Geometry check sheet. Reference: drawing and pictorial views, mm from the part's lowest x, y, z. A direction names the side the tool comes from. Coordinates: 2 decimals unless noted, no trailing zeros. Loops run counter-clockwise (first coordinate to the right, second up) from the corner with the lowest first, then second, coordinate; pieces in that order, holes last. Notation, with made-up numbers: M 22,-27.5 L 60,-27.5 A18 cw 60,-17.5 Z; hole C 51.5,-7.75 d9. An arc over 180 degrees is marked long. Write each question's results on one line, items separated by ' | '. Start each with the question number.
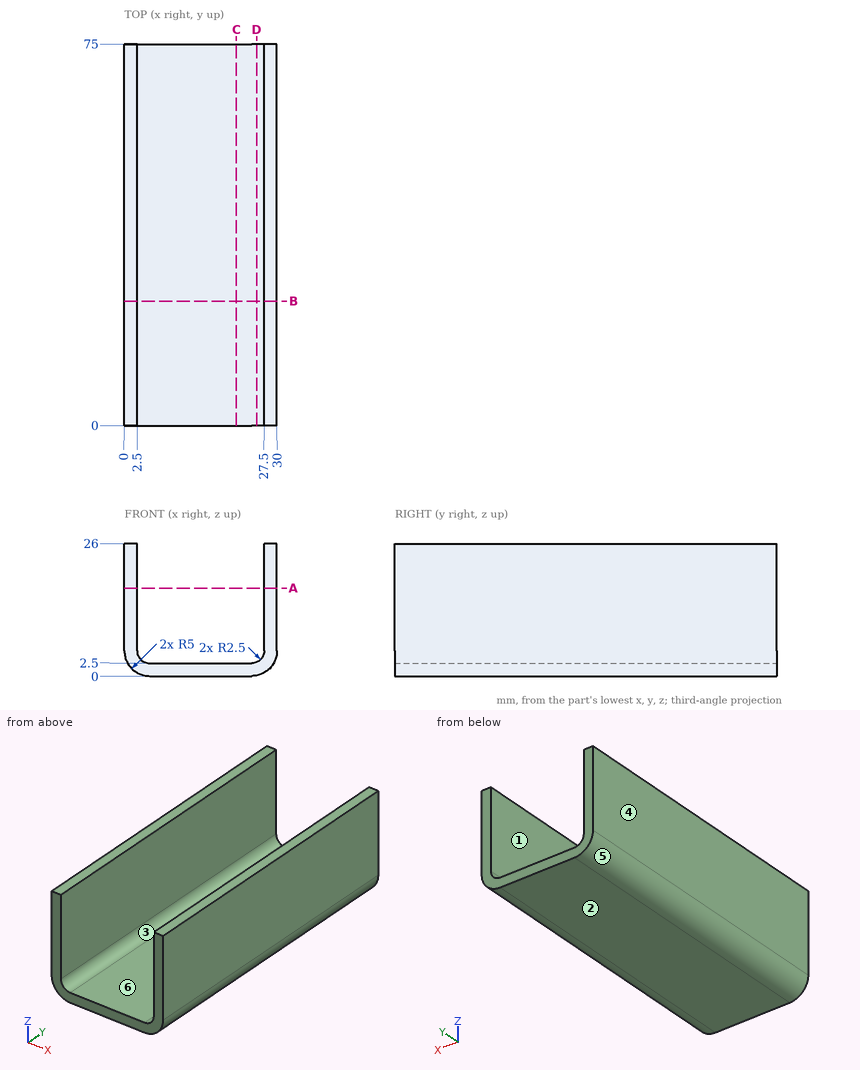
1) Set-up check for the marked faces 5 and 6: record each of +Z, -Z, +X, -X, +Y, -Y from which the full face is reachable in a straight line by a thin tool's end or side.
2) Thickness scan on probe 1 along X at (y, z) = (38.5, 13.75); probe 2 along Z at (x, y) = (8.5, 19); probe 3 along X at (y, z) = (47, 1). Record the ranges inside material, lowest first.
3) Release check for a two-part mould opening along X. For the marked faces 1, 2, 3 and 4 record: +X half, -X half, draft (parallel to the pull), parting line (faces both ways), or undercut.
4) Section check B-B (y = 24.5). Enter the section's corners in (x, z), then the cut area to 3 significant figures.
5) Section check A-A (z = 17.25). Enter the section's corners in (x, y).
6) Gauge pin test, flat end, axial feed: P1, Ø6, axis at x = 7.5, z = 9, coming from the +Y side. Record the tip position at first contact, or that the pin passes through.
7) Section check C-C (x = 22). Enter the section's corners in (y, z), then the cut area to 4 significant figures.
8) Section check D-D (x = 26). Enter the section's corners in (y, z).
Return value:
1) face 5: -Z, -X, +Y, -Y | face 6: +Z, +Y, -Y
2) probe 1: x = 0 to 2.5, 27.5 to 30 | probe 2: z = 0 to 2.5 | probe 3: x = 2 to 28
3) face 1: undercut | face 2: draft | face 3: undercut | face 4: -X half
4) outline: M 0,5 A5 ccw 5,0 L 25,0 A5 ccw 30,5 L 30,26 L 27.5,26 L 27.5,5 A2.5 cw 25,2.5 L 5,2.5 A2.5 cw 2.5,5 L 2.5,26 L 0,26 Z | area: 184 mm2
5) outline: M 0,0 L 2.5,0 L 2.5,75 L 0,75 Z; M 27.5,0 L 30,0 L 30,75 L 27.5,75 Z
6) P1: passes through
7) outline: M 0,0 L 75,0 L 75,2.5 L 0,2.5 Z | area: 187.5 mm2
8) outline: M 0,0.1 L 75,0.1 L 75,2.71 L 0,2.71 Z
